Print and shaded views of the part. All mm, measured from the part's lowest x, y and z. A direction names the side the tool comes from. Coordinates: 2 decimals unless noted, no trailing zeros. Order: outer loops, then holes, each group sorted by start corner. A loop starts at its lowest first (then second) coordinate and runs counter-clockwise, first axis right, second up. Notation, with made-up numbers: (-34.75, 37.25) -> (-29.75, 37.25) arc R33 ccw to (-29.75, 72.25) -> close; hole circle Ø5 at (-1, -12). An arc over 180 degrees is marked (long way). Write item = value, one per line. Start each with the question number.
Q1. Mould opens along Z. For the marked faces 1, 2, 3 and 4 say: +Z half, -Z half, draft (parallel to the pull), parting line (faces both ways), or undercut.
Q2. Cut at B-B, the plane y = 15. List the corners of the cut face in (x, z), plus the area to 3 significant figures.
Q3. Flat gauge pins, fed straight in: pin 1 (1.2 mm diameter, centred on x = 1.5, y = 1.5, fed in from +Z); pin 2 (5 mm diameter, centred on y = 23, z = 9.5, fed in from -X); pin 3 (2 mm diameter, centred on x = 2.5, y = 10.5, fed in from +Z). Where does each tip first touch, or does it go through?
Q4. Wall check: line 1 (Z direction, x = 0.95, y = 14); line 2 (Y direction, x = 0.55, z = 6.75) (1 decimal); line 3 (Z direction, x = 1.45, y = 7.5). Give the ranges that are in metal, low to high. Write a range as from..to.
Q5. 3-axis set-ups, long thin cutter, end or side, ignore diameter. For the marked faces 5, 6 and 7: which of +Z, -Z, +X, -X, +Y, -Y reach the whole face in a straight line?
Q6. Cut at A-A, the plane x = 0.9. List the corners of the cut face in (y, z) (1 decimal), plus the area to 3 significant figures.
Q7. Cut at C-C, the plane z = 4.5. List the corners of the cut face in (x, y).
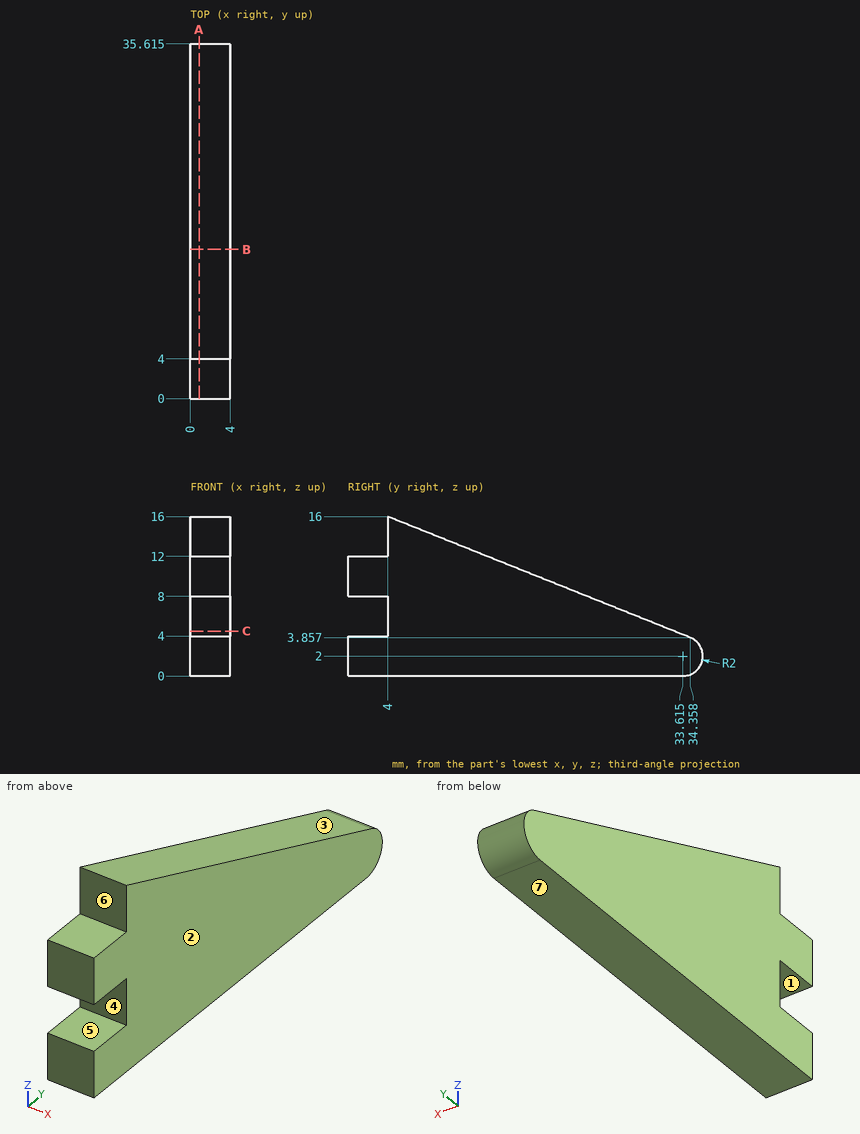
Here are the results:
q1.face_1 = undercut
q1.face_2 = draft
q1.face_3 = +Z half
q1.face_4 = undercut
q2.outline = (0, 0) -> (4, 0) -> (4, 11.6) -> (0, 11.6) -> close
q2.area = 46.4 mm²
q3.pin_1 = 12
q3.pin_2 = 0
q3.pin_3 = 13.8
q4.line_1 = 0..12
q4.line_2 = 4..27.1
q4.line_3 = 0..14.6
q5.face_5 = +X, -X, -Y
q5.face_6 = +Z, +X, -X, -Y
q5.face_7 = -Z, +X, -X, +Y, -Y
q6.outline = (0, 0) -> (33.6, 0) arc R2 ccw to (34.4, 3.9) -> (4, 16) -> (4, 12) -> (0, 12) -> (0, 8) -> (4, 8) -> (4, 4) -> (0, 4) -> close
q6.area = 337 mm²
q7.outline = (0, 4) -> (4, 4) -> (4, 32.75) -> (0, 32.75) -> close
